Read the model definition and answer for the solid it produces. Units are mm, in the model's axes. A direction names the side the tool comes from. Coordinates: 2 decimals unless noted, no trailing zeros. Loops run counter-clockwise (first coordinate to the right, second up) from the corner with the lowest first, then second, coordinate; pieces in that order, holes last. Notation, with made-up numbers: M -22.5,59 L -1.5,59 A18 ccw -1.5,91 Z; hole C 50,25 d6. An arc over 180 degrees is marked long. One line per item, written item: value. Start each with the question number.
```python
from build123d import *

# Parameters (mm, degrees)
F0_W     = 16
F0_H     = 16
F1_DEPTH = 16
F2_R     = 2
F3_DEPTH = 1
F4_R     = 2
F6_DEPTH = 1.27


with BuildPart() as f1:
    # F0 (on Front) → F1 (new body)
    with BuildSketch(Plane.XZ):
        with Locations((-24.35377, -4.09623)):
            Rectangle(F0_W, F0_H)
    extrude(amount=F1_DEPTH)

    # F2 (on face) → F3 (cut)
    with BuildSketch(Plane(origin=(0, 0, 0), x_dir=(-1, 0, 0), z_dir=(0, 1, 0))):
        with Locations((24.35377, -4.09623)):
            Circle(F2_R)
    extrude(amount=-F3_DEPTH, mode=Mode.SUBTRACT)

    # F4 (on face) → F6 (cut)
    with BuildSketch(Plane(origin=(-32.35377, 0, 0), x_dir=(0, -1, 0), z_dir=(-1, 0, 0))):
        with Locations((13, -9.09623)):
            Circle(F4_R)
        with Locations((3, 0.90377)):
            Circle(F4_R)
    extrude(amount=-F6_DEPTH, mode=Mode.SUBTRACT)


solid = f1.part
```
1) Consider line 1 along Z through (x, y) = (-31.7, -13); line 2 along Z through (x, y) = (-31.55, -3); line 3 along Y through (x, z) = (-23.5, -5.25). Determine where each line is inside the solid, lowest interval first.
2) For a pull along X with two mould halves and no side action, classify faces 4 (the face through (-22.356, -0.493, -4.008)), 5 (the face through (-16.354, -8, -4)), 6 (the face through (-32.354, -8, -4)), 7 (the face through (-24, -16, -4)) as released by +X, released by -X, zero draft, split by the parting line, or undercut.
3) A flat-ended cylindrical pin translates along its axis: pin 1 (1.2 mm diameter, centred on x = -24, z = -3.5, fed in from +Y). Find the tip coordinate at first contact, or state that the pin passes through.
4) Section A-A (y = -13) is taken. Determine the outline of the cut face in (x, z).
5) Section B-B (z = 0) is taken. Determine the outline of the cut face in (x, y).
6) A tool of negligible diameter and unlimited length cuts with its end or side. For faces 1 (the face through (-31.084, -3, 1)), 2 (the face through (-24, -1, -4)), 3 (the face through (-24, -8, 3.904)), from which of +Z, -Z, +X, -X, +Y, -Y can it reach the whole face along a straight path? Write none if from no direction.
Results found:
1. line 1: z = -12.1 to -11.1, -7.1 to 3.9
1. line 2: z = -12.1 to -1.1, 2.9 to 3.9
1. line 3: y = -16 to -1
2. face 4: undercut
2. face 5: released by +X
2. face 6: released by -X
2. face 7: zero draft
3. pin 1: stops at y = -1
4. outline: M -32.35,-12.1 L -16.35,-12.1 L -16.35,3.9 L -32.35,3.9 L -32.35,-7.1 L -31.08,-7.1 L -31.08,-11.1 L -32.35,-11.1 Z
5. outline: M -32.35,-16 L -16.35,-16 L -16.35,0 L -32.35,0 L -32.35,-1.22 L -31.08,-1.22 L -31.08,-4.78 L -32.35,-4.78 Z
6. face 1: -X
6. face 2: +Y
6. face 3: +Z, +X, -X, +Y, -Y
